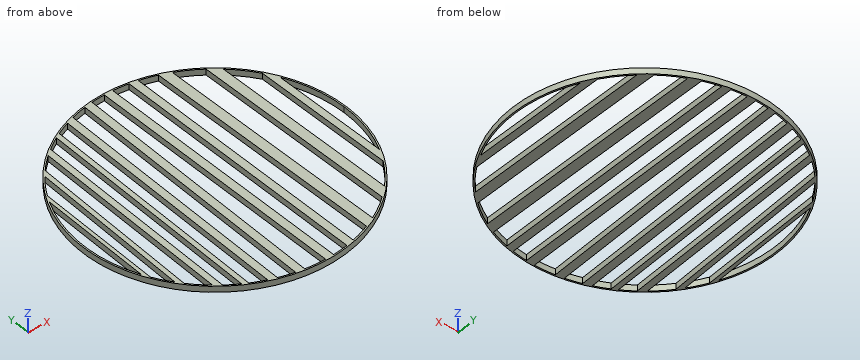
from build123d import *

# Parameters (mm, degrees)
F1_DEPTH = 20


with BuildPart() as f1:
    # F0 (on Top) → F1 (new body)
    with BuildSketch(Plane.XY):
        with BuildLine():
            Line((-270.5386970375, -346.9997311313), (-270.7217620056, -353.178039488))
            ThreePointArc((-270.7217620056, -353.178039488), (-250.9562000988, -367.4860346081), (-230.4360952891, -380.6891198707))
            Line((-230.4360952891, -380.6891198707), (-230.265657339, -374.9369641023))
            ThreePointArc((-230.2656573389, -374.9369641023), (-250.7914922543, -361.5295664436), (-270.5386970375, -346.9997311313))
        make_face()
        with BuildLine():
            ThreePointArc((-402.562994487, -177.6035908131), (-397.2206510106, -189.250507029), (-391.5414264828, -200.7369207392))
            Line((-391.5414264828, -200.7369207392), (-378.8101580312, 223.8366908537))
            ThreePointArc((-378.8101580312, 223.8366908537), (-385.1674232463, 212.7112034422), (-391.1980296982, 201.4053166136))
            Line((-391.1980296982, 201.4053166136), (-402.562994487, -177.6035908131))
        make_face()
        with BuildLine():
            ThreePointArc((-356.5130720875, -257.8728939433), (-349.3185745571, -267.5379103406), (-341.8621362052, -277.0023101514))
            Line((-341.8621362052, -277.0023101514), (-316.4372711676, 305.7244730407))
            ThreePointArc((-316.4372711676, 305.7244730407), (-324.6896849683, 296.9454638064), (-332.6986262228, 287.9437863707))
            Line((-332.6986262228, 287.9437863707), (-356.5130720875, -257.8728939433))
        make_face()
        with BuildLine():
            ThreePointArc((-290.771309932, -330.2302913429), (-280.7802245685, -338.7660925938), (-270.5386970375, -346.9997311313))
            Line((-270.5386970375, -346.9997311313), (-249.5187169425, 362.4091746843))
            ThreePointArc((-249.5187169425, 362.4091746843), (-260.22977901, 354.7963671127), (-270.708728898, 346.8670986105))
            Line((-270.708728898, 346.8670986105), (-290.771309932, -330.2302913429))
        make_face()
        with BuildLine():
            Line((-207.6622074156, 387.912886627), (-230.265657339, -374.9369641023))
            ThreePointArc((-230.2656573389, -374.9369641023), (-222.1173118779, -379.8208785258), (-213.8654246951, -384.5277364768))
            Line((-213.8654246951, -384.5277364768), (-190.7228909108, 396.5157990328))
            ThreePointArc((-190.7228909108, 396.5157990328), (-199.2389875692, 392.3057810336), (-207.6622074156, 387.912886627))
        make_face()
        with BuildLine():
            Line((-70.8738586956, 434.2544140865), (-70.7405367429, 439.341298379))
            ThreePointArc((-70.7405367429, 439.341298379), (-431.4752027521, 108.8767624889), (-270.7217620056, -353.178039488))
            Line((-270.7217620056, -353.178039488), (-270.5386970375, -346.9997311313))
            ThreePointArc((-270.5386970375, -346.9997311313), (-280.7802245685, -338.7660925938), (-290.771309932, -330.2302913429))
            ThreePointArc((-290.771309932, -330.2302913429), (-317.4343613856, -304.6890648049), (-341.8621362052, -277.0023101514))
            ThreePointArc((-341.8621362052, -277.0023101514), (-349.3185745571, -267.5379103406), (-356.5130720875, -257.8728939433))
            ThreePointArc((-356.5130720875, -257.8728939433), (-375.1166659405, -229.9727960731), (-391.5414264828, -200.7369207392))
            ThreePointArc((-391.5414264828, -200.7369207392), (-397.2206510106, -189.250507029), (-402.562994487, -177.6035908131))
            ThreePointArc((-402.562994487, -177.6035908131), (-439.8023179294, 13.187916588), (-391.1980296982, 201.4053166136))
            ThreePointArc((-391.1980296982, 201.4053166136), (-385.1674232463, 212.7112034422), (-378.8101580312, 223.8366908537))
            ThreePointArc((-378.8101580312, 223.8366908537), (-357.1954891114, 256.9268038926), (-332.6986262228, 287.9437863707))
            ThreePointArc((-332.6986262228, 287.9437863707), (-324.6896849683, 296.9454638064), (-316.4372711676, 305.7244730407))
            ThreePointArc((-316.4372711676, 305.7244730407), (-294.2928562808, 327.0958800445), (-270.708728898, 346.8670986105))
            ThreePointArc((-270.708728898, 346.8670986105), (-260.22977901, 354.7963671127), (-249.5187169425, 362.4091746843))
            ThreePointArc((-249.5187169425, 362.4091746843), (-228.9458652825, 375.7443156856), (-207.6622074156, 387.912886627))
            ThreePointArc((-207.6622074156, 387.912886627), (-199.2389875692, 392.3057810336), (-190.7228909108, 396.5157990328))
            ThreePointArc((-190.7228909108, 396.5157990328), (-169.0852127848, 406.2144640673), (-146.9564772982, 414.7334008494))
            ThreePointArc((-146.9564772982, 414.7334008494), (-134.2564645291, 419.0169468317), (-121.4318768159, 422.9116920741))
            ThreePointArc((-121.4318768159, 422.9116920741), (-96.3199787859, 429.3279185968), (-70.8738586956, 434.2544140865))
        make_face()
        with BuildLine():
            Line((-143.4181009985, -415.9702493039), (-121.4318768159, 422.9116920741))
            ThreePointArc((-121.4318768159, 422.9116920741), (-134.2564645291, 419.0169468317), (-146.9564772982, 414.7334008494))
            Line((-146.9564772982, 414.7334008494), (-168.4792645982, -406.4661577554))
            ThreePointArc((-168.4792645982, -406.4661577554), (-156.0210678261, -411.4090742733), (-143.4181009985, -415.9702493039))
        make_face()
        with BuildLine():
            ThreePointArc((-43.616286433, 437.8328671511), (-57.2730273731, 436.2565762662), (-70.8738586956, 434.2544140865))
            Line((-70.8738586956, 434.2544140865), (-93.5236465706, -429.9457262634))
            ThreePointArc((-93.5236465706, -429.9457262634), (-80.0463646466, -432.6575776603), (-66.4909418972, -434.9470710852))
            Line((-66.4909418972, -434.9470710852), (-43.616286433, 437.8328671511))
        make_face()
        with BuildLine():
            Line((0, 440), (0, -440))
            ThreePointArc((0, -440), (14.0186355194, -439.7766226827), (28.0230371971, -439.1067175372))
            Line((28.0230371971, -439.1067175372), (28.0230371971, 439.1067175372))
            ThreePointArc((28.0230371971, 439.1067175372), (14.0186355194, 439.7766226827), (0, 440))
        make_face()
        with BuildLine():
            Line((78.35839003, 432.9664683459), (78.35839003, -432.9664683459))
            ThreePointArc((78.35839003, -432.9664683459), (91.7286409393, -430.3322628289), (105.0109050122, -427.2852792088))
            Line((105.0109050122, -427.2852792088), (105.0109050122, 427.2852792088))
            ThreePointArc((105.0109050122, 427.2852792088), (91.7286409393, 430.3322628289), (78.35839003, 432.9664683459))
        make_face()
        with BuildLine():
            Line((158.8886932936, 410.3101060704), (167.7992454591, -406.7473579796))
            ThreePointArc((167.7992454591, -406.7473579796), (184.9665523772, -399.233483693), (201.798344937, -390.9954321737))
            Line((201.798344937, -390.9954321737), (193.2232359584, 395.3034038378))
            ThreePointArc((193.2232359584, 395.3034038378), (176.2157852134, 403.1724160228), (158.8886932936, 410.3101060704))
        make_face()
        with BuildLine():
            Line((268.376457209, 348.6747441613), (275.9167800325, -342.7388663348))
            ThreePointArc((275.9167800325, -342.7388663348), (292.9545944223, -328.2949978402), (309.2374568684, -313.0051042228))
            Line((309.2374568684, -313.0051042228), (302.3376646701, 319.6747355075))
            ThreePointArc((302.3376646701, 319.6747355075), (285.7252217666, 334.6058840583), (268.376457209, 348.6747441613))
        make_face()
        with BuildLine():
            Line((367.9772639554, 241.2317002633), (373.1507016006, -233.1492095096))
            ThreePointArc((373.1507016006, -233.1492095096), (385.3711791661, -212.3418335329), (396.4325833067, -190.8958011398))
            Line((396.4325833067, -190.8958011398), (392.175101476, 199.4960896417))
            ThreePointArc((392.175101476, 199.4960896417), (380.6486174495, 220.6957861714), (367.9772639554, 241.2317002633))
        make_face()
        with BuildLine():
            ThreePointArc((0, -445), (314.662517628, -314.662517628), (445, 0))
            ThreePointArc((445, 0), (288.570148447, 338.7510434306), (-70.7405367429, 439.341298379))
            Line((-70.7405367429, 439.341298379), (-70.8738586956, 434.2544140865))
            ThreePointArc((-70.8738586956, 434.2544140865), (-57.2730273731, 436.2565762662), (-43.616286433, 437.8328671511))
            ThreePointArc((-43.616286433, 437.8328671511), (-21.835045838, 439.4578828207), (0, 440))
            ThreePointArc((0, 440), (14.0186355194, 439.7766226827), (28.0230371971, 439.1067175372))
            ThreePointArc((28.0230371971, 439.1067175372), (53.2792424848, 436.7623178804), (78.35839003, 432.9664683459))
            ThreePointArc((78.35839003, 432.9664683459), (91.7286409393, 430.3322628289), (105.0109050122, 427.2852792088))
            ThreePointArc((105.0109050122, 427.2852792088), (132.2224966571, 419.663211847), (158.8886932936, 410.3101060704))
            ThreePointArc((158.8886932936, 410.3101060704), (176.2157852134, 403.1724160228), (193.2232359584, 395.3034038378))
            ThreePointArc((193.2232359584, 395.3034038378), (231.9744105691, 373.8821643795), (268.376457209, 348.6747441613))
            ThreePointArc((268.376457209, 348.6747441613), (285.7252217666, 334.6058840583), (302.3376646701, 319.6747355075))
            ThreePointArc((302.3376646701, 319.6747355075), (337.4445929766, 282.3670424658), (367.9772639554, 241.2317002633))
            ThreePointArc((367.9772639554, 241.2317002633), (380.6486174495, 220.6957861714), (392.175101476, 199.4960896417))
            ThreePointArc((392.175101476, 199.4960896417), (427.8767606738, 102.5742544467), (440, 0))
            ThreePointArc((440, 0), (428.969892099, -97.9021535643), (396.4325833067, -190.8958011398))
            ThreePointArc((396.4325833067, -190.8958011398), (385.3711791661, -212.3418335329), (373.1507016006, -233.1492095096))
            ThreePointArc((373.1507016006, -233.1492095096), (343.5224020131, -274.9406468952), (309.2374568684, -313.0051042228))
            ThreePointArc((309.2374568684, -313.0051042228), (292.9545944223, -328.2949978402), (275.9167800325, -342.7388663348))
            ThreePointArc((275.9167800325, -342.7388663348), (240.0731330091, -368.7341736362), (201.798344937, -390.9954321737))
            ThreePointArc((201.798344937, -390.9954321737), (184.9665523772, -399.233483693), (167.7992454591, -406.7473579796))
            ThreePointArc((167.7992454591, -406.7473579796), (136.7910673332, -418.1963700199), (105.0109050122, -427.2852792088))
            ThreePointArc((105.0109050122, -427.2852792088), (91.7286409393, -430.3322628289), (78.35839003, -432.9664683459))
            ThreePointArc((78.35839003, -432.9664683459), (53.2792424848, -436.7623178804), (28.0230371971, -439.1067175372))
            ThreePointArc((28.0230371971, -439.1067175372), (14.0186355194, -439.7766226827), (0, -440))
            Line((0, -440), (0, -445))
        make_face()
        with BuildLine():
            ThreePointArc((-230.4360952891, -380.6891198707), (-119.6209464466, -428.6208454698), (0, -445))
            Line((0, -445), (0, -440))
            ThreePointArc((0, -440), (-33.3413311259, -438.7349491877), (-66.4909418972, -434.9470710852))
            ThreePointArc((-66.4909418972, -434.9470710852), (-80.0463646466, -432.6575776603), (-93.5236465706, -429.9457262634))
            ThreePointArc((-93.5236465706, -429.9457262634), (-118.6767728932, -423.693077092), (-143.4181009985, -415.9702493039))
            ThreePointArc((-143.4181009985, -415.9702493039), (-156.0210678261, -411.4090742733), (-168.4792645982, -406.4661577554))
            ThreePointArc((-168.4792645982, -406.4661577554), (-191.4867852876, -396.1474612568), (-213.8654246951, -384.5277364768))
            ThreePointArc((-213.8654246951, -384.5277364768), (-222.1173118779, -379.8208785258), (-230.2656573389, -374.9369641023))
            Line((-230.265657339, -374.9369641023), (-230.4360952891, -380.6891198707))
        make_face()
    extrude(amount=-F1_DEPTH)


solid = f1.part
Design review of the part built by this model. Coordinates are the model's own, in mm. Coordinates: 2 decimals unless noted, no trailing zeros. Order: outer loops, then holes, each group sorted by start corner. A loop starts at its lowest first (then second) coordinate and runs counter-clockwise, first axis right, second up. Notation, with made-up numbers: (10, 85.25) - (66, 85.25) arc R25 cw to (66, 99.25) - close; hole circle Ø3 at (8.25, -8.5). An arc over 180 degrees is marked (long way). Put each result on its own line as item: value.
1) Take a section at A-A, the plane x = 220. Give the boundary of the cut face in (y, z), and give its area (3 significant figures).
Response values:
outline: (-386.81, -20) - (-381.05, -20) - (-381.05, 0) - (-386.81, 0) - close; (381.05, -20) - (386.81, -20) - (386.81, 0) - (381.05, 0) - close
area: 231 mm²
2) Insertion check: P1, Ø6, axis at y = -12.5, z = -11, coming from the +X side; P2, Ø12, axis at x = 157, y = -157.5, coming from the -Z side; P3, Ø12, axis at y = 343, z = -6.5, coming from the +X side; P4, Ø3, axis at y = 255.5, z = -9.5, coming from the -X side. Each pin has a flat end and moves straight along its axis. Give the tip position at first contact, or say it passes through.
Response values:
P1: stops at x = 444.9
P2: passes through
P3: stops at x = 290.61
P4: stops at x = -365.39
3) Wall thickness on L1, parallel to X at y = 397.5, z = -11; L2, parallel to Y at x = 218, z = -10.5; L3, parallel to Y at x = 71, z = -3: over which ranges is each line inside the solid? List them lowest first. Write a range as from..to.
Response values:
L1: x = -200.05..-188.66, -147.41..-122.1, -71.84..-44.67, 0..28.02, 78.36..105.01, 159.03..200.05
L2: y = -387.94..-382.2, 382.2..387.94
L3: y = -439.3..-434.23, 434.23..439.3
4) Take a section at B-B, the plane y = 51. Count the separate pieces of the cut face and the enclosed holes in it, and give its area (3 significant figures).
Response values:
separate pieces: 13
enclosed holes: 0
area: 5,470 mm²
5) Take a section at C-C, the plane x = 57.5. Give the boundary of the cut face in (y, z), and give its area (3 significant figures).
Response values:
outline: (-441.27, -20) - (-436.23, -20) - (-436.23, 0) - (-441.27, 0) - close; (436.23, -20) - (441.27, -20) - (441.27, 0) - (436.23, 0) - close
area: 202 mm²
